Model file for the job. Use its own axes, mm. A direction names the side the tool comes from. Give positions to 0.01 mm unless a question says otherwise; leave off trailing zeros. Write each loop counter-clockwise with the first axis right and the second up, starting at its lowest first coordinate (ties: lowest second). Pieces come first, ordered by that corner, then holes.
```python
from build123d import *

# Parameters (mm, degrees)
SKETCH1_R           = 2.1
BOSS_EXTRUDE1_DEPTH = 3


with BuildPart() as part:
    # Sketch1 → Boss-Extrude1 (new body)
    with BuildSketch(Plane.XY):
        with BuildLine():
            Line((-6.3, 110.8), (-3, 110.8))
            ThreePointArc((-3, 110.8), (-0.878679656, 109.921320344), (0, 107.8))
            Line((0, 107.8), (0, 9.2))
            ThreePointArc((0, 9.2), (-0.878679656, 7.078679656), (-3, 6.2))
            Line((-3, 6.2), (-6.3, 6.2))
            ThreePointArc((-6.3, 6.2), (-10.684062043, 4.384062043), (-12.5, 0))
            Line((-12.5, 0), (-12.5, -49))
            Line((-12.5, -49), (-9.5, -49))
            ThreePointArc((-9.5, -49), (-8.085786438, -49.585786438), (-7.5, -51))
            Line((-7.5, -51), (-7.5, -59))
            Line((-7.5, -59), (48, -59))
            Line((48, -59), (48, -0.5))
            Line((48, -0.5), (44, -0.5))
            Line((44, -0.5), (44, 8.5))
            Line((44, 8.5), (48, 8.5))
            Line((48, 8.5), (48, 114.5))
            Line((48, 114.5), (44, 114.5))
            Line((44, 114.5), (44, 123.2))
            Line((44, 123.2), (-6.3, 123.2))
            ThreePointArc((-6.3, 123.2), (-12.5, 117), (-6.3, 110.8))
        make_face()
        Circle(SKETCH1_R, mode=Mode.SUBTRACT)
        with Locations((0, 117)):
            Circle(SKETCH1_R, mode=Mode.SUBTRACT)
    extrude(amount=BOSS_EXTRUDE1_DEPTH)


solid = part.part
```
1. Probe probe 1 along Y at (x, z) = (44.5, 2.3); probe 2 along X at (y, z) = (10.5, 2.55); probe 3 along Y at (x, z) = (-3.5, 0.5). List the from-to ranges inside material, lowest first.
Calculated:
probe 1: y = -59 to -0.5, 8.5 to 114.5
probe 2: x = 0 to 48
probe 3: y = -59 to 6.2, 110.8 to 123.2
2. Slice it at B-B, the plane z = 2.15. Write the cut outline in (x, y), and give its area (3 significant figures).
Calculated:
outline: (-12.5, -49) - (-9.5, -49) arc R2 cw to (-7.5, -51) - (-7.5, -59) - (48, -59) - (48, -0.5) - (44, -0.5) - (44, 8.5) - (48, 8.5) - (48, 114.5) - (44, 114.5) - (44, 123.2) - (-6.3, 123.2) arc R6.2 ccw to (-6.3, 110.8) - (-3, 110.8) arc R3 cw to (0, 107.8) - (0, 9.2) arc R3 cw to (-3, 6.2) - (-6.3, 6.2) arc R6.2 ccw to (-12.5, 0) - close; hole circle Ø4.2 at (0, 0); hole circle Ø4.2 at (0, 117)
area: 9,550 mm2
3. Which spindle directions (+Z, -Z, +X, -X, +Y, -Y) get a long thin tool onto all of the face, cutting with end or side? Do faces 1 (the cylindrical face through (-0.9, 109.94, 1.48)), 2 (the flat face through (-7.5, -55, 1)), 3 (the flat face through (46, -0.5, 1)). Say none if no direction does.
Calculated:
face 1: +Z, -Z, -X
face 2: +Z, -Z, -X, -Y
face 3: +Z, -Z, +X
4. Slice it at A-A, the plane y = 117. Write the cut outline in (x, z), and give its area (3 significant figures).
Calculated:
outline: (-12.5, 0) - (-2.1, 0) - (-2.1, 3) - (-12.5, 3) - close; (2.1, 0) - (44, 0) - (44, 3) - (2.1, 3) - close
area: 157 mm2
5. Pull direction Y, two halves, no side cores. Call faces 4 (the flat face through (17, 33, 0)), 5 (the cylindrical face through (-0.86, 7.1, 1.48)), 6 (the flat face through (20, -59, 1)), 7 (the flat face through (19, 123.2, 1)): +Y half, -Y half, draft (parallel to the pull), parting line (faces both ways), or undercut.
Calculated:
face 4: draft
face 5: undercut
face 6: -Y half
face 7: +Y half
6. Pin check, flat tips, straight feed: P1, Ø0.9, axis at x = -11, z = 1, coming from the -Y side; P2, Ø1.5, axis at x = 46, z = 2, coming from the +Y side. Stop position of each tip, or through.
Calculated:
P1: stops at y = -49
P2: stops at y = 114.5
